Source: three-view drawing plus pictorial views. Frame: mm from the lowest corner of the part. A direction names the side the tool comes from. Give positions to 0.01 mm unless a question says otherwise; leave off trailing zeros. Order: outer loops, then holes, each group sorted by start corner. A loop starts at its lowest first (then second) coordinate and runs counter-clockwise, first axis right, second up. Notation, with made-up numbers: (47.25, -37.5) - (61.25, -37.5) arc R22 ccw to (61.25, 0.5) - close; hole circle Ø9 at (-10.75, -23.5). An arc over 180 degrees is marked (long way). Use CSV: the item, a comma, the result in double quotes.
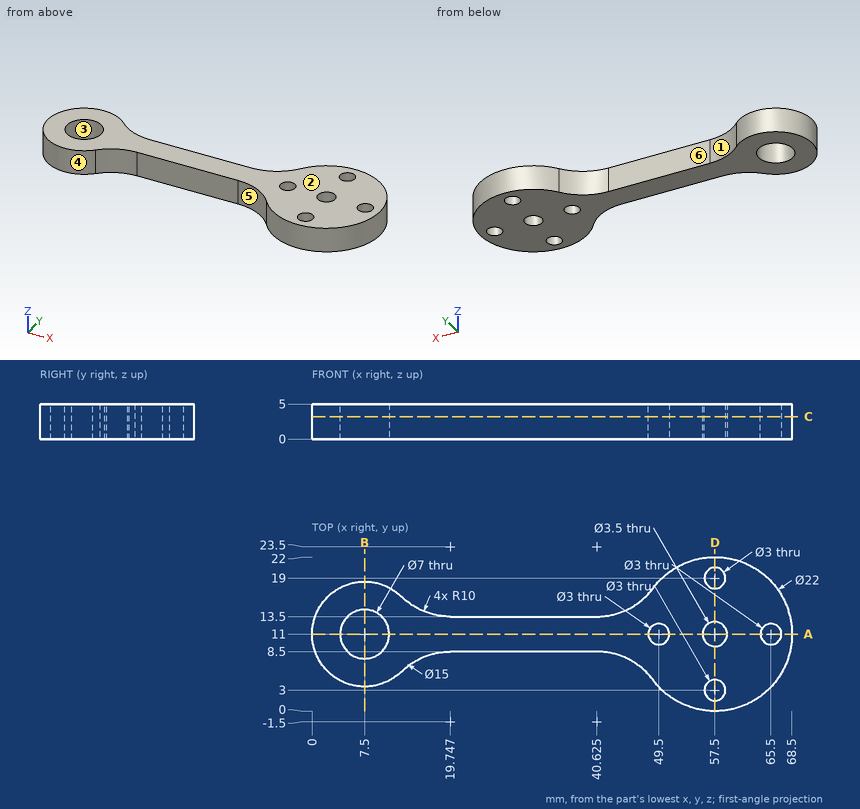
Item 1: Set-up query: the marked faces 4, 5 and 6. Return all of +Z, -Z, +X, -X, +Y, -Y with unobstructed straight access to the full face (end or side cutting, diameter ignored); none if empty.
Filled in:
face 4,"+Z, -Z"
face 5,"+Z, -Z, -Y"
face 6,"+Z, -Z, +Y"
Item 2: Section B-B on x = 7.5. Return the cut outline in (y, z), then the cut area to 3 significant figures.
Filled in:
outline,"(3.5, 0) - (7.5, 0) - (7.5, 5) - (3.5, 5) - close; (14.5, 0) - (18.5, 0) - (18.5, 5) - (14.5, 5) - close"
area,"40.0 mm2"
Item 3: Section A-A on y = 11. Return the cut outline in (x, z), then the cut area to 3 significant figures.
Filled in:
outline,"(0, 0) - (4, 0) - (4, 5) - (0, 5) - close; (11, 0) - (48, 0) - (48, 5) - (11, 5) - close; (51, 0) - (55.75, 0) - (55.75, 5) - (51, 5) - close; (59.25, 0) - (64, 0) - (64, 5) - (59.25, 5) - close; (67, 0) - (68.5, 0) - (68.5, 5) - (67, 5) - close"
area,"260 mm2"
Item 4: First-contact query: pin 1 (6.5 mm diameter, centred on x = 7.5, y = 11, fed in from +Z); pin 2 (2.5 mm diameter, centred on x = 32, z = 3, fed in from +Y); pin 3 (1.5 mm diameter, centred on x = 26.5, z = 3, fed in from -Y); pin 4 (3 mm diameter, centred on y = 6, z = 2, fed in from +X). Flat tips, straight axial feed; report the tip coordinate or a pass-through.
Filled in:
pin 1,"passes through"
pin 2,"stops at y = 13.5"
pin 3,"stops at y = 8.5"
pin 4,"stops at x = 67.93"
Item 5: Section D-D on x = 57.5. Return the cut outline in (y, z).
Filled in:
outline,"(0, 0) - (1.5, 0) - (1.5, 5) - (0, 5) - close; (4.5, 0) - (9.25, 0) - (9.25, 5) - (4.5, 5) - close; (12.75, 0) - (17.5, 0) - (17.5, 5) - (12.75, 5) - close; (20.5, 0) - (22, 0) - (22, 5) - (20.5, 5) - close"
Item 6: Material intervals for line 1 (Y direction, x = 57.5, z = 2.1); line 2 (Y direction, x = 7.5, z = 1.8); line 3 (Y direction, x = 65.5, z = 2.2), sorted ascending. Write a range as from..to.
Filled in:
line 1,"y = 0..1.5, 4.5..9.25, 12.75..17.5, 20.5..22"
line 2,"y = 3.5..7.5, 14.5..18.5"
line 3,"y = 3.45..9.5, 12.5..18.55"
Item 7: Mould query, pull axis Y, two halves, no side actions, for the marked faces 1, 2 and 3. Classes: released by +Y, released by -Y, zero draft, split by the parting line, or undercut.
Filled in:
face 1,"released by +Y"
face 2,"zero draft"
face 3,"undercut"
Item 8: Section C-C on z = 3.2. Count the separate pieces of the cut face and the enclosed holes in it, then the cut area to 3 significant figures.
Filled in:
separate pieces,"1"
enclosed holes,"6"
area,"656 mm2"
